Geometry check sheet. Reference: the model listing, model coordinates, mm. A direction names the side the tool comes from. Give positions to 0.01 mm unless a question says otherwise; leave off trailing zeros. Write each loop counter-clockwise with the first axis right and the second up, starting at its lowest first coordinate (ties: lowest second). Pieces come first, ordered by that corner, then holes. Notation, with made-up numbers: M -3,70.25 L 32,70.25 A17 ccw 32,83.25 Z; hole C 87,32.25 d3. An arc over 180 degrees is marked long. Use one line per item in the form item = value. Start each with the question number.
```python
from build123d import *

# Parameters (mm, degrees)
PAD_DEPTH       = 30
SKETCH003_R     = 5
HOLE_DEPTH      = 44
HOLE_TIPS_R     = 5
SKETCH005_R     = 2.5
HOLE001_DEPTH   = 60.001
SKETCH011_R     = 3.2
HOLE002_DEPTH   = 60
HOLE002_TIPS_R  = 3.2
SKETCH013_R     = 1.25
HOLE003_DEPTH   = 10
HOLE003_TIPS_R  = 1.25
SKETCH014_R     = 3.4
HOLE004_DEPTH   = 20
HOLE004_TIPS_R  = 3.4
SKETCH015_R     = 10
SKETCH015_R_2   = 3.5
SKETCH015_W     = 112.5
SKETCH015_H     = 5
POCKET001_DEPTH = 5
SKETCH016_R     = 1.6
HOLE005_DEPTH   = 20
HOLE005_TIPS_R  = 1.6
SKETCH029_R     = 2.75
POCKET007_DEPTH = 60.001


with BuildPart() as part:
    # Sketch → Revolution (revolve)
    with BuildSketch(Plane.XZ):
        Polygon((6, 60), (6.75, 30), (0, 30), (0, 60), align=None)
    revolve(axis=Axis((0, 0, 0), (0, 0, 1)))

    # Sketch006 → Pad (new body)
    with BuildSketch(Plane.XY):
        Polygon((0, 17.5), (62.5, 17.5), (62.5, -17.5), (0, -17.5), (-17.5, -17.5), (-17.5, 17.5), align=None)
    extrude(amount=PAD_DEPTH)

    # Sketch003 → Hole (cut)
    with BuildSketch(Plane.XY.offset(60)):
        Circle(SKETCH003_R)
    extrude(amount=-HOLE_DEPTH, mode=Mode.SUBTRACT)

    # Hole tips → Hole tip 1 section 0
    with BuildSketch(Plane.XY.offset(16), mode=Mode.PRIVATE) as hole_tip_1_s0:
        Circle(HOLE_TIPS_R)
    loft([hole_tip_1_s0.sketch, Vertex(0, 0, 12.995697)], mode=Mode.SUBTRACT)

    # Sketch005 → Hole001 (cut, through all)
    with BuildSketch(Plane.XY):
        with Locations((-2.5, 0)):
            Circle(SKETCH005_R)
    extrude(amount=HOLE001_DEPTH, mode=Mode.SUBTRACT)

    # Sketch011 → Hole002 (cut)
    with BuildSketch(Plane.YZ.offset(62.5)):
        with Locations((0, 20)):
            Circle(SKETCH011_R)
    extrude(amount=-HOLE002_DEPTH, mode=Mode.SUBTRACT)

    # Hole002 tips → Hole002 tip 1 section 0
    with BuildSketch(Plane.YZ.offset(2.5), mode=Mode.PRIVATE) as hole002_tip_1_s0:
        with Locations((0, 20)):
            Circle(HOLE002_TIPS_R)
    loft([hole002_tip_1_s0.sketch, Vertex(0.577246, 0, 20)], mode=Mode.SUBTRACT)

    # Sketch012 → Groove (revolve, cut)
    with BuildSketch(Plane.YZ.offset(45)):
        Polygon((15, 30), (15, 29), (12.9, 29), (12.9, 27.5), (10.4, 27.5), (10.4, 27.9), (10, 27.9), (10, 11.5), (5.4, 11.5), (4.788889, 6.5), (2.5, 6.5), (2.5, 0), (0, 0), (0, 30), align=None)
    revolve(axis=Axis((45, 0, 0), (0, 0, 1)), mode=Mode.SUBTRACT)

    # Sketch013 → Hole003 (cut)
    with BuildSketch(Plane.XY.offset(30)):
        with Locations((33.25, 13.75)):
            Circle(SKETCH013_R)
        with Locations((56.75, 13.75)):
            Circle(SKETCH013_R)
        with Locations((33.25, -13.75)):
            Circle(SKETCH013_R)
        with Locations((56.75, -13.75)):
            Circle(SKETCH013_R)
    extrude(amount=-HOLE003_DEPTH, mode=Mode.SUBTRACT)

    # Hole003 tips → Hole003 tip 1 section 0
    with BuildSketch(Plane.XY.offset(20), mode=Mode.PRIVATE) as hole003_tip_1_s0:
        with Locations((33.25, 13.75)):
            Circle(HOLE003_TIPS_R)
    loft([hole003_tip_1_s0.sketch, Vertex(33.25, 13.75, 19.248924)], mode=Mode.SUBTRACT)

    # Hole003 tips → Hole003 tip 2 section 0
    with BuildSketch(Plane.XY.offset(20), mode=Mode.PRIVATE) as hole003_tip_2_s0:
        with Locations((56.75, 13.75)):
            Circle(HOLE003_TIPS_R)
    loft([hole003_tip_2_s0.sketch, Vertex(56.75, 13.75, 19.248924)], mode=Mode.SUBTRACT)

    # Hole003 tips → Hole003 tip 3 section 0
    with BuildSketch(Plane.XY.offset(20), mode=Mode.PRIVATE) as hole003_tip_3_s0:
        with Locations((33.25, -13.75)):
            Circle(HOLE003_TIPS_R)
    loft([hole003_tip_3_s0.sketch, Vertex(33.25, -13.75, 19.248924)], mode=Mode.SUBTRACT)

    # Hole003 tips → Hole003 tip 4 section 0
    with BuildSketch(Plane.XY.offset(20), mode=Mode.PRIVATE) as hole003_tip_4_s0:
        with Locations((56.75, -13.75)):
            Circle(HOLE003_TIPS_R)
    loft([hole003_tip_4_s0.sketch, Vertex(56.75, -13.75, 19.248924)], mode=Mode.SUBTRACT)

    # Sketch014 → Hole004 (cut)
    with BuildSketch(Plane.YZ.offset(62.5)):
        with Locations((0, 20)):
            Circle(SKETCH014_R)
    extrude(amount=-HOLE004_DEPTH, mode=Mode.SUBTRACT)

    # Hole004 tips → Hole004 tip 1 section 0
    with BuildSketch(Plane.YZ.offset(42.5), mode=Mode.PRIVATE) as hole004_tip_1_s0:
        with Locations((0, 20)):
            Circle(HOLE004_TIPS_R)
    loft([hole004_tip_1_s0.sketch, Vertex(40.457074, 0, 20)], mode=Mode.SUBTRACT)

    # Sketch015 → Pocket001 (cut)
    with BuildSketch(Plane.XY.offset(4.5)):
        with Locations((45, 0)):
            Circle(SKETCH015_R)
        with Locations((45, 0)):
            Circle(SKETCH015_R_2, mode=Mode.SUBTRACT)
        with Locations((6.25, 15)):
            Rectangle(SKETCH015_W, SKETCH015_H)
        with Locations((6.25, -15)):
            Rectangle(SKETCH015_W, SKETCH015_H)
    extrude(amount=-POCKET001_DEPTH, mode=Mode.SUBTRACT)

    # Sketch016 → Hole005 (cut)
    with BuildSketch(Plane.YZ.offset(62.5)):
        with Locations((-12.5, 10)):
            Circle(SKETCH016_R)
        with Locations((12.5, 10)):
            Circle(SKETCH016_R)
    extrude(amount=-HOLE005_DEPTH, mode=Mode.SUBTRACT)

    # Hole005 tips → Hole005 tip 1 section 0
    with BuildSketch(Plane.YZ.offset(42.5), mode=Mode.PRIVATE) as hole005_tip_1_s0:
        with Locations((-12.5, 10)):
            Circle(HOLE005_TIPS_R)
    loft([hole005_tip_1_s0.sketch, Vertex(41.538623, -12.5, 10)], mode=Mode.SUBTRACT)

    # Hole005 tips → Hole005 tip 2 section 0
    with BuildSketch(Plane.YZ.offset(42.5), mode=Mode.PRIVATE) as hole005_tip_2_s0:
        with Locations((12.5, 10)):
            Circle(HOLE005_TIPS_R)
    loft([hole005_tip_2_s0.sketch, Vertex(41.538623, 12.5, 10)], mode=Mode.SUBTRACT)

    # Sketch029 → Pocket007 (cut, through all)
    with BuildSketch(Plane.XY):
        with Locations((25, 7.5)):
            Circle(SKETCH029_R)
    extrude(amount=POCKET007_DEPTH, mode=Mode.SUBTRACT)


solid = part.part
```
(1) Sectioned sample at C-C, the plane x = 45. State how many separate pieces and enclosed holes the cut face has, plus the area to 3 significant figures.
(2) Draft check along Z on faces 1 (the flat face through (22, 15, 4.5)), 2 (the cylindrical face through (47.44, -0.54, 3.2)), 3 (the cylindrical face through (19.909, -0.694, 16.876)), 4 (the flat face through (4, 4, 60)). Enter one of: released by +Z, released by -Z, zero draft, split by the parting line, or undercut.
(3) Depth check by flat-ended pin: pin 1 (3 mm diameter, centred on x = 33.25, y = 13.75, fed in from +Z); pin 2 (2 mm diameter, centred on x = 56.75, y = -13.75, fed in from +Z); pin 3 (10.5 mm diameter, centred on x = 43, y = 5, fed in from +Z). Enter the tip coordinate at first touch or a pass-through.
(4) Thickness scan on probe 1 along Y at (x, z) = (45, 28); probe 2 along Z at (x, y) = (30, 16); probe 3 along Z at (x, y) = (23, 0). Record the ranges inside material, lowest first. Write a range as [from, to].
(5) Tool access check on faces 5 (the conical face through (41.69, 12.47, 10.25)), 6 (the flat face through (22, -12.5, 2)), 7 (the cylindrical face through (33.922, 14.804, 25.07)). Record the directions out of +Z, -Z, +X, -X, +Y, -Y that give a thin tool (end or side, any length) a straight path to the whole face; none if there is none.
(6) Sectioned sample at A-A, the plane z = 14.5. Record the boundary of the cut face in (x, y), plus the area to 3 significant figures.
(7) Sectioned sample at D-D, the plane z = 22. Record the boundary of the cut face in (x, y), plus the area to 3 significant figures.
(8) Sectioned sample at B-B, the plane y = 8.5. Record the boundary of the cut face in (x, z).
Numbers:
q1.separate_pieces = 2
q1.enclosed_holes = 2
q1.area = 459 mm2
q2.face_1 = released by -Z
q2.face_2 = zero draft
q2.face_3 = undercut
q2.face_4 = released by +Z
q3.pin_1 = 30
q3.pin_2 = 19.85
q3.pin_3 = 27.9
q4.probe_1 = [-17.5, -12.9], [12.9, 17.5]
q4.probe_2 = [4.5, 30]
q4.probe_3 = [0, 16.8], [23.2, 30]
q5.face_5 = +X
q5.face_6 = -Z, +X, -X, -Y
q5.face_7 = +Z
q6.outline = M -17.5,-17.5 L 62.5,-17.5 L 62.5,17.5 L -17.5,17.5 Z; hole M -1.25,-2.17 A2.5 ccw long -1.25,2.17 A2.5 ccw long Z; hole C 25,7.5 d5.5; hole C 45,0 d20
q6.area = 2,430 mm2
q7.outline = M -17.5,-17.5 L 62.5,-17.5 L 62.5,-2.75 L 54.61,-2.75 A10 cw 35.32,-2.5 L 4.33,-2.5 A5 cw long 4.33,2.5 L 35.32,2.5 A10 cw 54.61,2.75 L 62.5,2.75 L 62.5,17.5 L -17.5,17.5 Z; hole C 25,7.5 d5.5; hole C 33.25,-13.75 d2.5; hole C 33.25,13.75 d2.5; hole C 56.75,-13.75 d2.5; hole C 56.75,13.75 d2.5
q7.area = 2,170 mm2
q8.outline = M -17.5,0 L 22.44,0 L 22.44,30 L -17.5,30 Z; M 27.56,0 L 39.73,0 L 39.73,4.5 L 50.27,4.5 L 50.27,0 L 62.5,0 L 62.5,30 L 57.36,30 L 57.36,29 L 54.7,29 L 54.7,27.5 L 50.99,27.5 L 50.99,27.9 L 50.27,27.9 L 50.27,11.5 L 39.73,11.5 L 39.73,27.9 L 39.01,27.9 L 39.01,27.5 L 35.3,27.5 L 35.3,29 L 32.64,29 L 32.64,30 L 27.56,30 Z
